Work out the finished part from the listing and answer in its coordinate system (mm). Face numbers are marked on the shaded views. A direction names the side the tool comes from. Round coordinates to 2 decimals unless told otherwise and drop trailing zeros. Write each loop counter-clockwise with the first axis right and the second up, starting at its lowest first coordinate (ties: lowest second). Pieces come first, ordered by that corner, then holes. Notation, with made-up numbers: (40, 69.25) - (75, 69.25) arc R21 cw to (75, 73.25) - close; hole circle Ø4 at (-3, 77). An arc over 180 degrees is marked (long way). Write item = value, one per line. Start each with the question number.
from build123d import *

# Parameters (mm, degrees)
F1_DEPTH  = 19.05
F4_DEPTH  = 19.05
F5_R      = 2.54
F9_DEPTH  = 1.27
F11_DEPTH = 1.27
F13_DEPTH = 1.27
F14_W     = 41.0627422772
F14_H     = 5.3488574922
F15_DEPTH = 22.606
F16_W     = 14.7093571723
F16_H     = 14.4864893518
F17_DEPTH = 6.35


# Not quite as in the source:
# - a feature of the source that left no trace in its solid (it failed there, or was rolled back) is left out


with BuildPart() as f1:
    # F0 (on Front) → F1 (new body)
    with BuildSketch(Plane.XZ):
        Polygon((0, 6.35), (0, 0), (49.7539146826, 0), (49.7539146826, 8.4803946126), (30.7039146826, 8.4803946126), (30.7039146826, 15.4774815776), (18.0039146826, 15.4774815776), (12.5200406866, 8.4803946126), align=None)
    extrude(amount=F1_DEPTH)

    # F2 (on face) + F3 (on face) → F4 (join)
    with BuildSketch(Plane.XZ.offset(19.05)):
        with BuildLine():
            ThreePointArc((4.1796790518, 0), (7.3546790518, -3.175), (10.5296790518, 0))
            Line((10.5296790518, 0), (4.1796790518, 0))
        make_face()
        with BuildLine():
            Line((4.1796790518, 0), (10.5296790518, 0))
            ThreePointArc((10.5296790518, 0), (7.3546790518, 3.175), (4.1796790518, 0))
        make_face()
    with BuildSketch(Plane.XZ.offset(19.05)):
        with BuildLine():
            ThreePointArc((38.9472560108, 0), (42.1222560108, -3.175), (45.2972560108, 0))
            Line((45.2972560108, 0), (38.9472560108, 0))
        make_face()
    extrude(amount=-F4_DEPTH)

    # F5
    f5_edges = [f1.edges().sort_by_distance(p)[0] for p in [
        (0, -9.525, 6.35),
    ]]
    fillet(f5_edges, radius=F5_R)

    # F8 (on face) → F9 (cut)
    with BuildSketch(Plane(origin=(0, 0, 0), x_dir=(-1, 0, 0), z_dir=(0, 1, 0))):
        with BuildLine():
            ThreePointArc((-10.5296790518, 0), (-7.3546790518, -3.175), (-4.1796790518, 0))
            ThreePointArc((-4.1796790518, 0), (-7.3546790518, 3.175), (-10.5296790518, 0))
        make_face()
    extrude(amount=-F9_DEPTH, mode=Mode.SUBTRACT)

    # F10 (on face) → F11 (cut)
    with BuildSketch(Plane(origin=(0, 0, 0), x_dir=(-1, 0, 0), z_dir=(0, 1, 0))):
        with BuildLine():
            ThreePointArc((-45.2972560108, 0), (-42.1222560108, -3.175), (-38.9472560108, 0))
            ThreePointArc((-38.9472560108, 0), (-42.1222560108, 3.175), (-45.2972560108, 0))
        make_face()
    extrude(amount=-F11_DEPTH, mode=Mode.SUBTRACT)

    # F12 (on face) → F13 (cut)
    with BuildSketch(Plane.XZ.offset(19.05)):
        with BuildLine():
            ThreePointArc((38.9472560108, 0), (42.1222560108, -3.175), (45.2972560108, 0))
            ThreePointArc((45.2972560108, 0), (42.1222560108, 3.175), (38.9472560108, 0))
        make_face()
        with BuildLine():
            ThreePointArc((4.1796790518, 0), (7.3546790518, -3.175), (10.5296790518, 0))
            ThreePointArc((10.5296790518, 0), (7.3546790518, 3.175), (4.1796790518, 0))
        make_face()
    extrude(amount=-F13_DEPTH, mode=Mode.SUBTRACT)

    # F14 (on face) → F15 (cut)
    with BuildSketch(Plane(origin=(0, 0, 0), x_dir=(1, 0, 0), z_dir=(0, 0, -1))):
        with Locations((24.7110501904, 9.5833707601)):
            Rectangle(F14_W, F14_H)
    extrude(amount=F15_DEPTH, mode=Mode.SUBTRACT)

    # F16 (on face) → F17 (cut)
    with BuildSketch(Plane.XY.offset(8.4803946126)):
        with Locations((39.8935656995, -9.6948046703)):
            Rectangle(F16_W, F16_H)
    extrude(amount=-F17_DEPTH, mode=Mode.SUBTRACT)


solid = f1.part
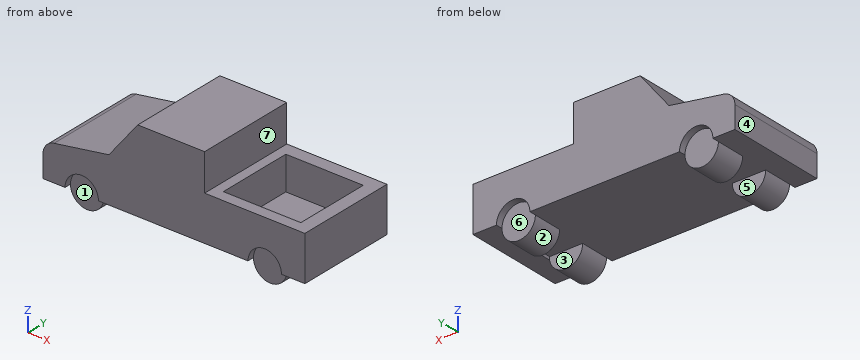
1. Each of these flat-tipped pins is pushed along its axis until it touches: pin 1 (10 mm diameter, centred on x = 8.5, y = -8, fed in from -Z) (3 decimals); pin 2 (1 mm diameter, centred on x = 42.5, z = -1.5, fed in from -Y); pin 3 (6 mm diameter, centred on x = 17.5, y = -3, fed in from -Z); pin 4 (1.5 mm diameter, centred on y = -8.5, z = 12.5, fed in from +X). Where does it stop, or does it pass through?
2. Find section A-A on y = -6. Give the vertices of the cut face in (x, z) (3 decimals).
3. Find section C-C on x = 43. Give the vertices of the cut face in (y, z).
4. Consider line 1 (Y direction, x = 36, z = 8.25); line 2 (X direction, y = -13.5, z = 3.5); line 3 (X direction, y = -15.75, z = -0.25). Determine where each line is inside the solid, lowest interval first.
5. Which of the six approach directions +Z, -Z, +X, -X, +Y, -Y give full straight-line access (tool end or side, diameter ignored) to the marked faces 5, 6 and 7?
6. Find section D-D on x = 22. Give the vertices of the cut face in (y, z), plus the area to 3 significant figures.
7. Find section B-B on x = 35. Give the vertices of the cut face in (y, z).
8. For a pull along X with two mould halves and no side action, classify the marked faces 1, 2, 3 and 4 as released by +X, released by -X, zero draft, split by the parting line, or undercut.
Answer key:
q1.pin_1 = -3.175
q1.pin_2 = -17.78
q1.pin_3 = 0
q1.pin_4 = 30.7
q2.outline = (0, 0) - (4.18, 0) arc R3.175 ccw to (10.53, 0) - (38.947, 0) arc R3.175 ccw to (45.297, 0) - (49.754, 0) - (49.754, 8.48) - (47.248, 8.48) - (47.248, 2.13) - (32.539, 2.13) - (32.539, 8.48) - (30.704, 8.48) - (30.704, 15.477) - (18.004, 15.477) - (12.52, 8.48) - (2.114, 6.71) arc R2.54 ccw to (0, 4.206) - close
q3.outline = (-19.05, 3.05) - (-17.78, 3.05) - (-17.78, -3.05) - (-12.26, -3.05) - (-12.26, 0) - (-6.91, 0) - (-6.91, -3.05) - (-1.27, -3.05) - (-1.27, 3.05) - (0, 3.05) - (0, 8.48) - (-2.45, 8.48) - (-2.45, 2.13) - (-16.94, 2.13) - (-16.94, 8.48) - (-19.05, 8.48) - close
q4.line_1 = -19.05 to -16.94, -2.45 to 0
q4.line_2 = 0 to 32.54, 47.25 to 49.75
q4.line_3 = 4.19 to 10.52, 38.96 to 45.29
q5.face_5 = -Z, -X
q5.face_6 = -Z, +Y
q5.face_7 = +Z, +X, +Y, -Y
q6.outline = (-19.05, 0) - (0, 0) - (0, 15.48) - (-19.05, 15.48) - close
q6.area = 295 mm²
q7.outline = (-19.05, 0) - (0, 0) - (0, 8.48) - (-2.45, 8.48) - (-2.45, 2.13) - (-16.94, 2.13) - (-16.94, 8.48) - (-19.05, 8.48) - close
q8.face_1 = undercut
q8.face_2 = undercut
q8.face_3 = zero draft
q8.face_4 = released by -X
